from build123d import *

# Parameters (mm, degrees)
SKETCH1_R           = 6.15
BOSS_EXTRUDE2_DEPTH = 4
SKETCH4_W           = 22
SKETCH4_H           = 8.5
CUT_EXTRUDE2_DEPTH  = 1
SKETCH5_R           = 1.6
CUT_EXTRUDE3_DEPTH  = 5


with BuildPart() as part:
    # Sketch1 → Boss-Extrude2 (new body)
    with BuildSketch(Plane(origin=(0, 0, 0), x_dir=(1, 0, 0), z_dir=(0, 1, 0))):
        with BuildLine():
            Line((10, -1.5), (32, -1.5))
            Line((32, -1.5), (32, -8.5))
            Line((32, -8.5), (32, -10))
            Line((32, -10), (10, -10))
            Line((10, -10), (10, -8.5))
            Line((10, -8.5), (0, -8.5))
            ThreePointArc((0, -8.5), (-8.5, 0), (0, 8.5))
            Line((0, 8.5), (10, 8.5))
            Line((10, 8.5), (10, -1.5))
        make_face()
        Circle(SKETCH1_R, mode=Mode.SUBTRACT)
    extrude(amount=BOSS_EXTRUDE2_DEPTH)

    # Sketch4 → Cut-Extrude2 (cut)
    with BuildSketch(Plane(origin=(0, 4, 0), x_dir=(1, 0, 0), z_dir=(0, 1, 0))):
        with Locations((21, -5.75)):
            Rectangle(SKETCH4_W, SKETCH4_H)
    extrude(amount=-CUT_EXTRUDE2_DEPTH, mode=Mode.SUBTRACT)

    # Sketch5 → Cut-Extrude3 (cut, through all)
    with BuildSketch(Plane.XZ):
        with Locations((17, 5.75)):
            Circle(SKETCH5_R)
        with Locations((25, 5.75)):
            Circle(SKETCH5_R)
    extrude(amount=-CUT_EXTRUDE3_DEPTH, mode=Mode.SUBTRACT)


solid = part.part
Here's how the part is built. I have some questions about the finished solid (model axes, mm). A direction names the side the tool comes from. Round coordinates to 2 decimals unless told otherwise and drop trailing zeros. Order: outer loops, then holes, each group sorted by start corner. A loop starts at its lowest first (then second) coordinate and runs counter-clockwise, first axis right, second up. Notation, with made-up numbers: M -19,-5 L -12,-5 A25 cw -12,28 Z; hole C 9.5,9 d8. An arc over 180 degrees is marked long. Return JSON: item names as keys, results as strings. Group by question number.
1. If we section it at C-C on y = 3.5: List the corners of the cut face in (x, z) for me, then the cut area to 3 significant figures.
2. If we section it at A-A on z = 0: List the corners of the cut face in (x, y) for me.
3. If we mould it in two halves opening along X, with no side actions, what happens to faces 4 (the face through (5, 2, 8.5)), 5 (the face through (23.73, 1.48, 4.78)), 6 (the face through (32, 1, 6))? For each: pulls with the +X half, pulls with the -X half, needs draft (parallel to the pull), parting line crosses it, or undercut.
4. I'm going to push flat-ended pins straight in: pin 1 Ø9.5 at (x, z) = (21, 8) entering from +Y; pin 2 Ø1.2 at (y, z) = (1.5, 9.5) entering from -X; pin 3 Ø3 at (x, z) = (17, 5.75) entering from -Y; pin 4 Ø1 at (y, z) = (0.5, -5) entering from -X. Where does each tip first touch, or does it pass through?
5. On a 3-axis mill with a long thin cutter (end or side, diameter ignored), from which of +Z, -Z, +X, -X, +Y, -Y can I reach the whole of each face in a straight line? I mean faces 1 (the face through (10, 1, 9)), 2 (the face through (21, 1, 1.5)), 3 (the face through (21, 3, 6)). Say none if no direction works.
6. If we section it at D-D on z = 5.75: List the corners of the cut face in (x, y) for me, then the cut area to 3 significant figures.
7. If we section it at B-B on x = 17: List the corners of the cut face in (y, z) for me.
8. Please list where these lines run through material, in increasing order: probe 1 along Z at (x, y) = (17, 2.45); probe 2 along Y at (x, z) = (21, 2.75); probe 3 along X at (y, z) = (2.15, 8.75).
Reply:
{
 "1": {"outline": "M 0,-8.5 L 10,-8.5 L 10,8.5 L 0,8.5 A8.5 ccw Z; hole C 0,0 d12.3", "area": "165 mm^2"},
 "2": {"outline": "M -8.5,0 L -6.15,0 L -6.15,4 L -8.5,4 Z; M 6.15,0 L 10,0 L 10,4 L 6.15,4 Z"},
 "3": {"face 4": "needs draft", "face 5": "undercut", "face 6": "pulls with the +X half"},
 "4": {"pin 1": "y = 3", "pin 2": "x = 10", "pin 3": "through", "pin 4": "x = -7.21"},
 "5": {"face 1": "+Z, -X, +Y, -Y", "face 2": "-Z, +X, +Y, -Y", "face 3": "+Z, -Z, +X, +Y"},
 "6": {"outline": "M -6.26,0 L -2.18,0 L -2.18,4 L -6.26,4 Z; M 2.18,0 L 15.4,0 L 15.4,3 L 10,3 L 10,4 L 2.18,4 Z; M 18.6,0 L 23.4,0 L 23.4,3 L 18.6,3 Z; M 26.6,0 L 32,0 L 32,3 L 26.6,3 Z", "area": "94.4 mm^2"},
 "7": {"outline": "M 0,1.5 L 3,1.5 L 3,4.15 L 0,4.15 Z; M 0,7.35 L 3,7.35 L 3,10 L 0,10 Z"},
 "8": {"probe 1": "1.5 to 4.15, 7.35 to 10", "probe 2": "0 to 3", "probe 3": "10 to 32"}
}
